from build123d import *

# Parameters (mm, degrees)
SKETCH_1_W          = 65
SKETCH_1_H          = 57
EXTRUDE_1_DEPTH     = 167
SKETCH_2_W          = 4
SKETCH_2_H          = 10
CUT_EXTRUDE_1_DEPTH = 10
SKETCH_3_W          = 65
SKETCH_3_H          = 57
EXTRUDE_2_DEPTH     = 1
SKETCH_4_W          = 4
SKETCH_4_H          = 10
CUT_EXTRUDE_2_DEPTH = 10


with BuildPart() as part:
    # Эскиз1 → Бобышка-Вытянуть1 (new body)
    with BuildSketch(Plane(origin=(0, 0, 0), x_dir=(0, 0, -1), z_dir=(1, 0, 0))):
        Rectangle(SKETCH_1_W, SKETCH_1_H)
        with BuildLine():
            Line((23.5, -24.5), (-23.5, -24.5))
            ThreePointArc((-23.5, -24.5), (-27.035533906, -23.035533906), (-28.5, -19.5))
            Line((-28.5, -19.5), (-28.5, 19.5))
            ThreePointArc((-28.5, 19.5), (-27.035533906, 23.035533906), (-23.5, 24.5))
            Line((-23.5, 24.5), (23.5, 24.5))
            ThreePointArc((23.5, 24.5), (27.035533906, 23.035533906), (28.5, 19.5))
            Line((28.5, 19.5), (28.5, -19.5))
            ThreePointArc((28.5, -19.5), (27.035533906, -23.035533906), (23.5, -24.5))
        make_face(mode=Mode.SUBTRACT)
    extrude(amount=-EXTRUDE_1_DEPTH)

    # Эскиз2 → Вырез-Вытянуть1 (cut)
    with BuildSketch(Plane.XY.offset(32.5)):
        with Locations((-3, -13.5)):
            Rectangle(SKETCH_2_W, SKETCH_2_H)
    extrude(amount=-CUT_EXTRUDE_1_DEPTH, mode=Mode.SUBTRACT)

    # Эскиз3 → Бобышка-Вытянуть2 (add)
    with BuildSketch(Plane.ZY.offset(167)):
        Rectangle(SKETCH_3_W, SKETCH_3_H)
    extrude(amount=EXTRUDE_2_DEPTH)

    # Эскиз4 → Вырез-Вытянуть2 (cut)
    with BuildSketch(Plane(origin=(0, 0, -32.5), x_dir=(-1, 0, 0), z_dir=(0, 0, -1))):
        with Locations((3, 13.5)):
            Rectangle(SKETCH_4_W, SKETCH_4_H)
    extrude(amount=-CUT_EXTRUDE_2_DEPTH, mode=Mode.SUBTRACT)


solid = part.part
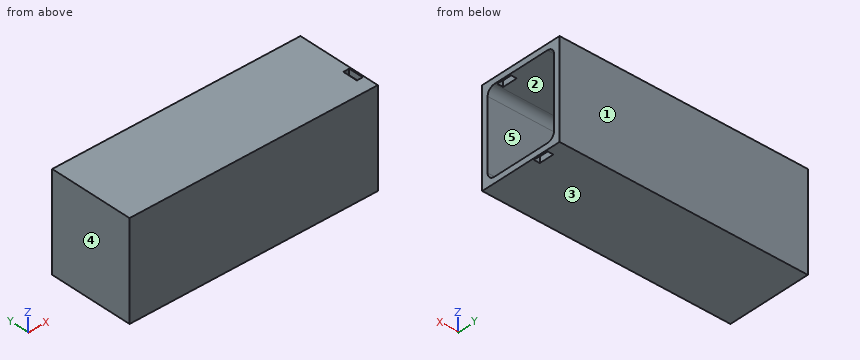
Work out the finished part from the listing and answer in its coordinate system (mm). Face numbers are marked on the shaded views. A direction names the side the tool comes from. Round coordinates to 2 decimals unless told otherwise and drop trailing zeros. Loops run counter-clockwise (first coordinate to the right, second up) from the corner with the lowest first, then second, coordinate; pieces in that order, holes last. Notation, with made-up numbers: (62.5, 73) - (102.5, 73) arc R16 ccw to (102.5, 92) - close; hole circle Ø7 at (-22, 31). An arc over 180 degrees is marked (long way). Use one line per item in the form item = value. Start each with the question number.
(1) Find section C-C on y = -6.5. Determine the outline of the cut face in (x, z).
(2) Determine the mould class of the marked faces 3, 4 and 5 for opening direction Z: +Z half, -Z half, draft (parallel to the pull), parting line (faces both ways), or undercut.
(3) Consider line 1 (Y direction, x = -85, z = 10.5); line 2 (Z direction, x = -7.5, y = -3); line 3 (X direction, y = -2, z = -27). Determine where each line is inside the solid, lowest interval first.
(4) Find section D-D on z = 14. Determine the outline of the cut face in (x, y).
(5) Which of the six approach directions +Z, -Z, +X, -X, +Y, -Y give full straight-line access (tool end or side, diameter ignored) to the marked faces 1 and 2?
(6) Flat-ended cylindrical pins translate along their axes: P1, Ø1.2, axis at y = -12.5, z = 30, coming from the +X side; P2, Ø5, axis at y = 19, z = -10, coming from the +X side. Find the tip coordinate at first contact, or state that the pin passes through.
(7) Find section A-A on y = -15. Determine the outline of the cut face in (x, z).
(8) Find section B-B on x = -12. Determine the outline of the cut face in (y, z), and give its area (3 significant figures).
Answer list:
q1.outline = (-168, -32.5) - (0, -32.5) - (0, -28.5) - (-167, -28.5) - (-167, 28.5) - (0, 28.5) - (0, 32.5) - (-168, 32.5) - close
q2.face_3 = -Z half
q2.face_4 = draft
q2.face_5 = undercut
q3.line_1 = -28.5 to -24.5, 24.5 to 28.5
q3.line_2 = -32.5 to -28.5, 28.5 to 32.5
q3.line_3 = -168 to -167
q4.outline = (-168, -28.5) - (0, -28.5) - (0, -24.5) - (-167, -24.5) - (-167, 24.5) - (0, 24.5) - (0, 28.5) - (-168, 28.5) - close
q5.face_1 = +Z, -Z, +X, -X, +Y
q5.face_2 = +X
q6.P1 = 0
q6.P2 = -167
q7.outline = (-168, -32.5) - (0, -32.5) - (0, -28.5) - (-167, -28.5) - (-167, 28.5) - (-5, 28.5) - (-5, 32.5) - (-168, 32.5) - close; (-1, 28.5) - (0, 28.5) - (0, 32.5) - (-1, 32.5) - close
q8.outline = (-28.5, -32.5) - (28.5, -32.5) - (28.5, 32.5) - (-28.5, 32.5) - close; hole (-24.5, -23.5) arc R5 ccw to (-19.5, -28.5) - (19.5, -28.5) arc R5 ccw to (24.5, -23.5) - (24.5, 23.5) arc R5 ccw to (19.5, 28.5) - (-19.5, 28.5) arc R5 ccw to (-24.5, 23.5) - close
q8.area = 933 mm^2
